Read the model definition and answer for the solid it produces. Units are mm, in the model's axes. A direction names the side the tool comes from. Round coordinates to 2 decimals unless told otherwise and drop trailing zeros. Write each loop counter-clockwise with the first axis right and the second up, starting at its lowest first coordinate (ties: lowest second). Pieces come first, ordered by that corner, then holes. Notation, with made-up numbers: (1.5, 15.25) -> (10.5, 15.25) arc R28 cw to (10.5, 33.25) -> close; hole circle Ø11 at (17.25, 88). An arc over 180 degrees is marked (long way). Return JSON: item names as keys, results as strings.
from build123d import *

# Parameters (mm, degrees)
SKETCH002_W      = 1
SKETCH002_H      = 1
EXTRUDE002_DEPTH = 9
SKETCH003_W      = 4
SKETCH003_H      = 1.4
EXTRUDE003_DEPTH = 0.5
SKETCH001_W      = 1.85
SKETCH001_H      = 1.4
EXTRUDE001_DEPTH = 8
SKETCH_W         = 3.2
SKETCH_H         = 2.54
EXTRUDE_DEPTH    = 8.5
CHAMFER_SIZE     = 0.4
ARRAY001_X_COUNT = 4
ARRAY001_X_PITCH = 2.54


with BuildPart() as extrude002:
    # Sketch002 → Extrude002 (new body)
    with BuildSketch(Plane.XY):
        Rectangle(SKETCH002_W, SKETCH002_H)
    extrude(amount=EXTRUDE002_DEPTH)


with BuildPart() as extrude003:
    # Sketch003 → Extrude003 (new body)
    with BuildSketch(Plane.XY):
        Rectangle(SKETCH003_W, SKETCH003_H)
    extrude(amount=EXTRUDE003_DEPTH)


with BuildPart() as fusion:
    # Sketch001 → Extrude001 (new body)
    with BuildSketch(Plane.XY):
        Rectangle(SKETCH001_W, SKETCH001_H)
    extrude(amount=EXTRUDE001_DEPTH)

    # Fusion: union Extrude002, Extrude003
    add(extrude002.part)
    add(extrude003.part)


with BuildPart() as body:
    # Sketch → Extrude (new body)
    with BuildSketch(Plane.XY):
        Rectangle(SKETCH_W, SKETCH_H)
    extrude(amount=EXTRUDE_DEPTH)

    # Cut001: cut Fusion
    add(fusion.part, mode=Mode.SUBTRACT)

    # Chamfer
    chamfer_edges = [body.edges().sort_by_distance(p)[0] for p in [
        (0.5, 0, 8.5),
        (0, 0.5, 8.5),
        (-0.5, 0, 8.5),
        (0, -0.5, 8.5),
    ]]
    chamfer(chamfer_edges, length=CHAMFER_SIZE)

    # Array001 X: body ×4


with BuildPart() as body_1:
    add(body.part)
    with Locations(*[(i * ARRAY001_X_PITCH, 0, 0) for i in range(1, ARRAY001_X_COUNT)]):
        add(body.part)


solid = body_1.part
Item 1: Straight lines are drawn through the part: L1, parallel to X at y = 0.35, z = 4.75 (3 decimals); L2, parallel to X at y = 0.25, z = 8.25; L3, parallel to Y at x = 5.5, z = 0.5. For each, find the intervals that lie inside material, in ascending order. Write a range as [from, to].
Worked answers:
{"L1": "x = [-1.6, -0.925], [0.925, 1.615], [3.465, 4.155], [6.005, 6.695], [8.545, 9.22]", "L2": "x = [-1.6, -0.65], [0.65, 1.89], [3.19, 4.43], [5.73, 6.97], [8.27, 9.22]", "L3": "y = [-1.27, -0.7], [0.7, 1.27]"}
Item 2: Flat-ended cylindrical pins translate along their axes: pin 1 (0.8 mm diameter, centred on x = 4, y = 0, fed in from -Z); pin 2 (0.7 mm diameter, centred on x = 2.5, y = -0.5, fed in from -Z). Find the tip coordinate at first contact, or state that the pin passes through.
Worked answers:
{"pin 1": "stops at z = 0.5", "pin 2": "stops at z = 0"}
Item 3: A tool of negligible diameter and unlimited length cuts with its end or side. For faces 1 (the flat face through (6.005, 0, 4)), 2 (the flat face through (9.22, 0, 4)), from which of +Z, -Z, +X, -X, +Y, -Y can it reach the whole face along a straight path? Write none if from no direction.
Worked answers:
{"face 1": "-Z", "face 2": "+Z, -Z, +X, +Y, -Y"}
Item 4: Section D-D (x = 7) is taken. Give the vertices of the cut face in (y, z).
Worked answers:
{"outline": "(-1.27, 0) -> (-0.7, 0) -> (-0.7, 8) -> (0.7, 8) -> (0.7, 0) -> (1.27, 0) -> (1.27, 8.5) -> (0.9, 8.5) -> (0.62, 8.22) -> (-0.62, 8.22) -> (-0.9, 8.5) -> (-1.27, 8.5) -> close"}
Item 5: Section C-C (y = -0.2) is taken. State how many separate pieces and enclosed holes the cut face has, then the cut area to 3 significant figures.
Worked answers:
{"separate pieces": "5", "enclosed holes": "0", "area": "28.4 mm2"}
Item 6: For a pull along Y with two mould halves and no side action, classify faces 3 (the flat face through (-1.6, 0, 4)), 4 (the flat face through (4, -1.27, 4)), 5 (the flat face through (-0.925, 0, 4)) as released by +Y, released by -Y, zero draft, split by the parting line, or undercut.
Worked answers:
{"face 3": "zero draft", "face 4": "released by -Y", "face 5": "undercut"}
Item 7: Section A-A (z = 4.25) is taken. Give the vertices of the cut face in (x, y) (3 decimals).
Worked answers:
{"outline": "(-1.6, -1.27) -> (9.22, -1.27) -> (9.22, 1.27) -> (-1.6, 1.27) -> close; hole (-0.925, -0.7) -> (0.925, -0.7) -> (0.925, 0.7) -> (-0.925, 0.7) -> close; hole (1.615, -0.7) -> (3.465, -0.7) -> (3.465, 0.7) -> (1.615, 0.7) -> close; hole (4.155, -0.7) -> (6.005, -0.7) -> (6.005, 0.7) -> (4.155, 0.7) -> close; hole (6.695, -0.7) -> (8.545, -0.7) -> (8.545, 0.7) -> (6.695, 0.7) -> close"}
Item 8: Section B-B (x = 2.5) is taken. Give the vertices of the cut face in (y, z).
Worked answers:
{"outline": "(-1.27, 0) -> (-0.7, 0) -> (-0.7, 8) -> (-0.5, 8) -> (-0.5, 8.1) -> (-0.9, 8.5) -> (-1.27, 8.5) -> close; (0.5, 8) -> (0.7, 8) -> (0.7, 0) -> (1.27, 0) -> (1.27, 8.5) -> (0.9, 8.5) -> (0.5, 8.1) -> close"}
